Verification items for this drawing (mm, ordinates from the low corner). Coordinates: 2 decimals unless noted, no trailing zeros. Loops run counter-clockwise (first coordinate to the right, second up) from the corner with the lowest first, then second, coordinate; pieces in that order, holes last. Notation, with made-up numbers: (45.5, 21.5) - (82.5, 21.5) arc R15 ccw to (82.5, 31.5) - close; hole circle Ø2 at (76, 73.25). An arc over 180 degrees is marked (long way). Write each question's results on one line, items separated by ' | '. Start each with the question number.
(1) Sectioned sample at A-A (z = 9.75). Enter the section's corners in (x, y).
(2) Sectioned sample at B-B (x = 257.5). Enter the section's corners in (y, z).
(3) Go/stop test with flat-tipped pins: pin 1 Ø6.5 at (x, y) = (200, 112.5) entering from +Z; pin 2 Ø3 at (y, z) = (220, 8.5) entering from -X. Record where each tip stops, or that it passes through.
(4) Material ranges on probe 1 along Y at (x, z) = (204.5, 12); probe 2 along Z at (x, y) = (206.5, 62), recorded low to high.
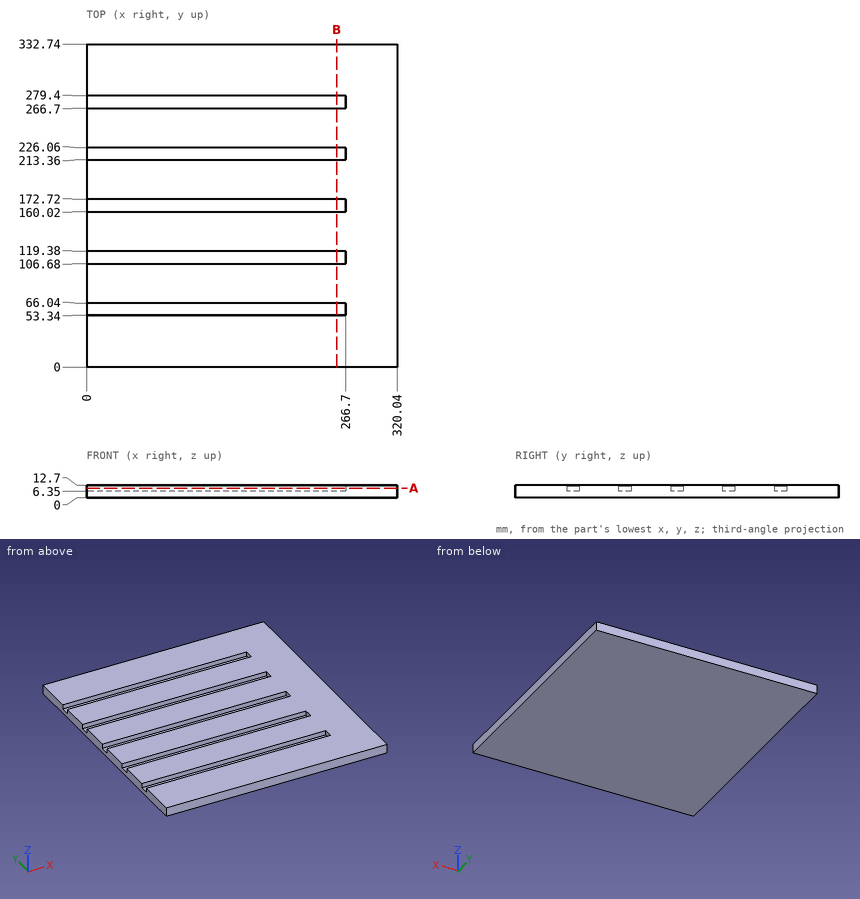
Outcome:
1) outline: (0, 0) - (320.04, 0) - (320.04, 332.74) - (0, 332.74) - (0, 279.4) - (266.7, 279.4) - (266.7, 266.7) - (0, 266.7) - (0, 226.06) - (266.7, 226.06) - (266.7, 213.36) - (0, 213.36) - (0, 172.72) - (266.7, 172.72) - (266.7, 160.02) - (0, 160.02) - (0, 119.38) - (266.7, 119.38) - (266.7, 106.68) - (0, 106.68) - (0, 66.04) - (266.7, 66.04) - (266.7, 53.34) - (0, 53.34) - close
2) outline: (0, 0) - (332.74, 0) - (332.74, 12.7) - (279.4, 12.7) - (279.4, 6.35) - (266.7, 6.35) - (266.7, 12.7) - (226.06, 12.7) - (226.06, 6.35) - (213.36, 6.35) - (213.36, 12.7) - (172.72, 12.7) - (172.72, 6.35) - (160.02, 6.35) - (160.02, 12.7) - (119.38, 12.7) - (119.38, 6.35) - (106.68, 6.35) - (106.68, 12.7) - (66.04, 12.7) - (66.04, 6.35) - (53.34, 6.35) - (53.34, 12.7) - (0, 12.7) - close
3) pin 1: stops at z = 6.35 | pin 2: stops at x = 266.7
4) probe 1: y = 0 to 53.34, 66.04 to 106.68, 119.38 to 160.02, 172.72 to 213.36, 226.06 to 266.7, 279.4 to 332.74 | probe 2: z = 0 to 6.35
